from build123d import *

# Parameters (mm, degrees)
F1_DEPTH = 351.282
F2_R     = 48.95754
F2_R_2   = 105.097299
F3_DEPTH = 1374.14


with BuildPart() as f1:
    # F0 (on Front) → F1 (new body)
    with BuildSketch(Plane.XZ):
        with BuildLine():
            ThreePointArc((391.798198, 58.458883), (173.454343, 122.011763), (-44.592593, 57.447519))
            ThreePointArc((-44.592593, 57.447519), (-281.676548, -26.572557), (-30.87141, -7.468691))
            ThreePointArc((-30.87141, -7.468691), (215.289624, -197.780053), (391.798198, 58.458883))
        make_face()
    extrude(amount=F1_DEPTH)

    # F2 (on face) → F3 (cut)
    with BuildSketch(Plane.XZ.offset(351.282)):
        with Locations((-174.473122, 38.385659)):
            Circle(F2_R)
        with Locations((185.898572, -5.635798)):
            Circle(F2_R_2)
    extrude(amount=-F3_DEPTH, mode=Mode.SUBTRACT)


solid = f1.part
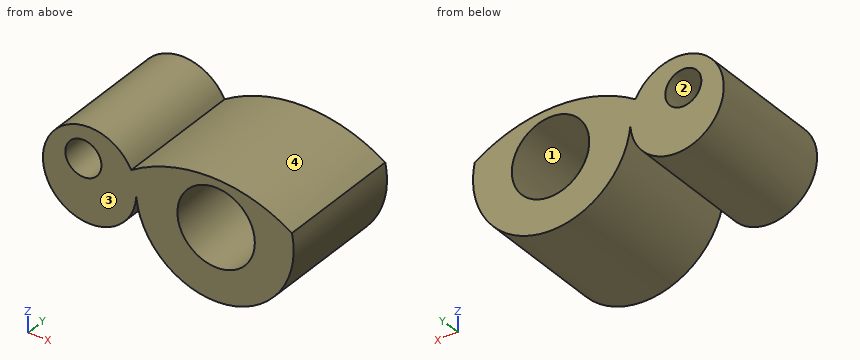
Verification items for the finished model (mm, model axes). Face numbers are marked on the shaded views. Coordinates: 2 decimals unless noted, no trailing zeros. Order: outer loops, then holes, each group sorted by start corner. A loop starts at its lowest first (then second) coordinate and runs counter-clockwise, first axis right, second up. Notation, with made-up numbers: M 82,78 L 116,78 A18 cw 116,84 Z; hole C -26,-11 d1. An arc over 180 degrees is marked long. Return JSON: item names as keys, results as strings.
1) Cross-section at B-B, the plane x = -195. Record the boundary of the cut face in (y, z).
Answer list:
{"outline": "M -351.28,-121.55 L 0,-121.55 L 0,-6.06 L -351.28,-6.06 Z; M -351.28,82.83 L 0,82.83 L 0,120.88 L -351.28,120.88 Z"}
2) Gauge pin test, flat ends, axial feed: pin 1 (2 mm diameter, centred on x = 93, y = -167.5, fed in from -Z); pin 2 (10 mm diameter, centred on y = -315.5, z = -141.5, fed in from -X); pin 3 (1.5 mm diameter, centred on y = -118, z = -44, fed in from -X). Record the tip position at first contact, or that the pin passes through.
Answer list:
{"pin 1": "z = -181.3", "pin 2": "x = 29.71", "pin 3": "x = -276.94"}
3) Cross-section at D-D, the plane z = 13.5. Record the boundary of the cut face in (x, y).
Answer list:
{"outline": "M -283.66,-351.28 L -216.63,-351.28 L -216.63,0 L -283.66,0 Z; M -132.31,-351.28 L 82.56,-351.28 L 82.56,0 L -132.31,0 Z; M 289.24,-351.28 L 396.49,-351.28 L 396.49,0 L 289.24,0 Z"}
4) Release check for a two-part mould opening along Z. For the marked faces 1, 2, 3 and 4 record: +Z half, -Z half, draft (parallel to the pull), parting line (faces both ways), or undercut.
Answer list:
{"face 1": "undercut", "face 2": "undercut", "face 3": "draft", "face 4": "+Z half"}
5) Thickness scan on L1, parallel to X at y = -308, z = -39.5; L2, parallel to X at y = -77, z = -25.5; L3, parallel to Z at x = 100, y = -316. Record the ranges inside material, lowest first. Write a range as [from, to].
Answer list:
{"L1": "[-278.22, -36.87], [-25.18, 86.41], [285.39, 389.73]", "L2": "[-281.9, -33.19], [-28.29, 82.7], [289.1, 392.84]", "L3": "[-183.91, -66.19], [54.92, 115.1]"}
6) Cross-section at C-C, the plane y = -169.5. Record the boundary of the cut face in (x, z), and give its area (3 significant figures).
Answer list:
{"outline": "M -44.59,57.45 A126.87 ccw long -30.87,-7.47 A214.21 ccw long 391.8,58.46 A403.64 ccw Z; hole C -174.47,38.39 d97.92; hole C 185.9,-5.64 d210.19", "area": "118,000 mm2"}
7) Cross-section at A-A, the plane z = -57. Record the boundary of the cut face in (x, y), and give its area (3 significant figures).
Answer list:
{"outline": "M -271.06,-351.28 L -44.03,-351.28 L -44.03,0 L -271.06,0 Z; M -19.87,-351.28 L 94.21,-351.28 L 94.21,0 L -19.87,0 Z; M 277.59,-351.28 L 384.43,-351.28 L 384.43,0 L 277.59,0 Z", "area": "157,000 mm2"}
